Geometry check sheet. Reference: drawing and pictorial views, mm from the part's lowest x, y, z. A direction names the side the tool comes from. Coordinates: 2 decimals unless noted, no trailing zeros. Write each loop counter-clockwise with the first axis right and the second up, starting at its lowest first coordinate (ties: lowest second). Pieces come first, ordered by that corner, then holes. Notation, with made-up numbers: (81, 68) - (112, 68) arc R22 ccw to (112, 82) - close; hole circle Ø1 at (16.5, -11). An arc over 180 degrees is marked (long way). Use one line per item in the form item = value. Start each with the question number.
(1) Sectioned sample at D-D (x = 95). Record the cut outline in (y, z).
(2) Sectioned sample at A-A (x = 49.5). Record the cut outline in (y, z).
(3) Tool access check on the marked faces 1 and 2. Record the directions out of +Z, -Z, +X, -X, +Y, -Y that give a thin tool (end or side, any length) a straight path to the whole face; none if there is none.
(4) Material ranges on line 1 (X direction, y = 50.8, z = 7.5); line 2 (X direction, y = 48, z = 10.75); line 3 (Y direction, x = 11.5, z = 15.5), recorded low to high. Write a range as [from, to].
(5) Gauge pin test, flat ends, axial feed: pin 1 Ø21.5 at (x, y) = (49, 55) entering from +Z; pin 2 Ø10 at (x, y) = (85, 16.5) entering from -Z; pin 3 Ø8 at (y, z) = (55.5, 17) entering from -X; pin 4 Ø9.5 at (x, z) = (46, 18.5) entering from +Y. Record the tip position at first contact, or that the pin passes through.
(6) Mould release check, pull along Y, two halves, no side actions. Record for the marked faces 3 and 4: released by +Y, released by -Y, zero draft, split by the parting line, or undercut.
(7) Sectioned sample at B-B (z = 6.25). Count the separate pieces of the cut face and the enclosed holes in it, and give its area (3 significant figures).
(8) Sectioned sample at C-C (y = 43). Record the cut outline in (x, z), and give its area (3 significant figures).
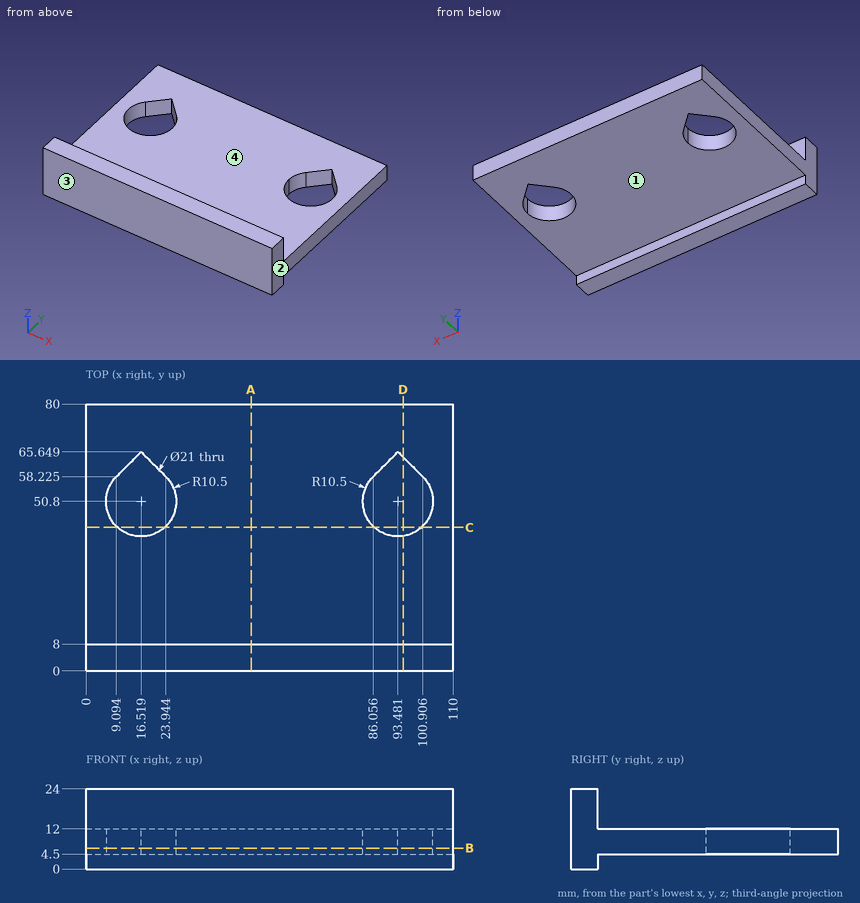
Answers below:
q1.outline = (0, 0) - (8, 0) - (8, 4.5) - (40.41, 4.5) - (40.41, 12) - (8, 12) - (8, 24) - (0, 24) - close; (64.13, 4.5) - (80, 4.5) - (80, 12) - (64.13, 12) - close
q2.outline = (0, 0) - (8, 0) - (8, 4.5) - (80, 4.5) - (80, 12) - (8, 12) - (8, 24) - (0, 24) - close
q3.face_1 = -Z, +X, -X, +Y
q3.face_2 = +Z, -Z, +X, +Y, -Y
q4.line_1 = [0, 6.02], [27.02, 82.98], [103.98, 110]
q4.line_2 = [0, 6.4], [26.64, 83.36], [103.6, 110]
q4.line_3 = [0, 8]
q5.pin_1 = 12
q5.pin_2 = 4.5
q5.pin_3 = through
q5.pin_4 = 8
q6.face_3 = released by -Y
q6.face_4 = zero draft
q7.separate_pieces = 1
q7.enclosed_holes = 2
q7.area = 8,060 mm2
q8.outline = (0, 4.5) - (9.49, 4.5) - (9.49, 12) - (0, 12) - close; (23.55, 4.5) - (86.45, 4.5) - (86.45, 12) - (23.55, 12) - close; (100.51, 4.5) - (110, 4.5) - (110, 12) - (100.51, 12) - close
q8.area = 614 mm2
